Model file for the job. Use its own axes, mm. A direction names the side the tool comes from. Round coordinates to 2 decimals unless told otherwise and drop trailing zeros. Order: outer loops, then holes, each group sorted by start corner. A loop starts at its lowest first (then second) coordinate and runs counter-clockwise, first axis right, second up. Notation, with made-up numbers: (-28.75, 26.25) -> (-22.75, 26.25) arc R31 cw to (-22.75, 57.25) -> close; hole circle Ø10 at (-17, 9.25). An arc over 180 degrees is marked (long way). Answer as CSV lines item,"result".
```python
from build123d import *

# Parameters (mm, degrees)
SKETCH1_R             = 3
BOSS_EXTRUDE1_DEPTH   = 2
SKETCH2_R             = 3
BOSS_EXTRUDE2_DEPTH   = 2
SKETCH3_R             = 5
CUT_EXTRUDE1_DEPTH    = 38
BOSS_EXTRUDE3_DEPTH   = 35
CUT_EXTRUDE2_DEPTH    = 13
SKETCH6_R             = 3.5
CUT_EXTRUDE3_DEPTH    = 42
SKETCH7_W             = 6
SKETCH7_H             = 6
CUT_EXTRUDE4_DEPTH    = 5
BODY_MOVE_COPY1_ANGLE = 90
BODY_MOVE_COPY2_ANGLE = 45
BODY_MOVE_COPY3_ANGLE = 45
CUT_EXTRUDE5_DEPTH    = 10
BOSS_EXTRUDE4_START   = 1
BOSS_EXTRUDE4_DEPTH   = 1


with BuildPart() as part:
    # Sketch1 → Boss-Extrude1 (new body)
    with BuildSketch(Plane.XY):
        with BuildLine():
            Line((10, 0), (10, 25))
            Line((10, 25), (10, 25.027864045))
            ThreePointArc((10, 25.027864045), (10.597396767, 27.130788493), (12.211145618, 28.605572809))
            Line((12.211145618, 28.605572809), (15, 30))
            Line((15, 30), (15, 60))
            Line((15, 60), (-9.181612248, 3.962069729))
            ThreePointArc((-9.181612248, 3.962069729), (-2.022854113, -9.793266117), (10, 0))
        make_face()
        Circle(SKETCH1_R, mode=Mode.SUBTRACT)
    extrude(amount=BOSS_EXTRUDE1_DEPTH)


with BuildPart() as body_2:
    # Sketch2 → Boss-Extrude2 (new body)
    with BuildSketch(Plane.XY.offset(8)):
        with BuildLine():
            Line((10, 0), (10, 25.027864045))
            Line((10, 25.027864045), (10, 25.043361255))
            ThreePointArc((10, 25.043361255), (10.602103374, 27.153882167), (12.22714926, 28.629027198))
            Line((12.22714926, 28.629027198), (15, 30))
            Line((15, 30), (15, 60))
            Line((15, 60), (-9.181612248, 3.962069729))
            ThreePointArc((-9.181612248, 3.962069729), (-2.022854113, -9.793266117), (10, 0))
        make_face()
        Circle(SKETCH2_R, mode=Mode.SUBTRACT)
    extrude(amount=BOSS_EXTRUDE2_DEPTH)


with BuildPart() as cut_extrude1_tool:
    # Sketch3 → Cut-Extrude1 (new body)
    with BuildSketch(Plane(origin=(0, 60, 0), x_dir=(1, 0, 0), z_dir=(0, 1, 0))):
        with Locations((15, -5)):
            Circle(SKETCH3_R)
    extrude(amount=-CUT_EXTRUDE1_DEPTH)


with BuildPart() as part_1:
    add(part.part)

    # Cut-Extrude1: cut by cut_extrude1_tool
    add(cut_extrude1_tool.part, mode=Mode.SUBTRACT)



with BuildPart() as body_2_1:
    add(body_2.part)

    # Cut-Extrude1: cut by cut_extrude1_tool
    add(cut_extrude1_tool.part, mode=Mode.SUBTRACT)


with BuildPart() as part_2:
    add(part_1.part)

    add(body_2_1.part)  # Boss-Extrude3 merges body 2
    # Sketch4 → Boss-Extrude3 (add)
    with BuildSketch(Plane(origin=(0, 60, 0), x_dir=(1, 0, 0), z_dir=(0, 1, 0))):
        with BuildLine():
            ThreePointArc((15, 0), (10, -5), (15, -10))
            Line((15, -10), (15, 0))
        make_face()
        with BuildLine():
            Line((15, 0), (15, -10))
            ThreePointArc((15, -10), (18.535533906, -8.535533906), (20, -5))
            ThreePointArc((20, -5), (18.535533906, -1.464466094), (15, 0))
        make_face()
    extrude(amount=-BOSS_EXTRUDE3_DEPTH)

    # Sketch5 → Cut-Extrude2 (cut)
    with BuildSketch(Plane.XY):
        with BuildLine():
            Line((10, 25.027864045), (10, 25.043361255))
            ThreePointArc((10, 25.043361255), (10.602103374, 27.153882167), (12.22714926, 28.629027198))
            Line((12.22714926, 28.629027198), (15, 30))
            Line((15, 30), (20, 32.472135955))
            Line((20, 32.472135955), (20, 25))
            Line((20, 25), (20, 22.63115285))
            Line((20, 22.63115285), (10, 22.63115285))
            Line((10, 22.63115285), (10, 25.027864045))
        make_face()
    extrude(amount=CUT_EXTRUDE2_DEPTH, mode=Mode.SUBTRACT)

    # Sketch6 → Cut-Extrude3 (cut)
    with BuildSketch(Plane(origin=(0, 60, 0), x_dir=(1, 0, 0), z_dir=(0, 1, 0))):
        with Locations(Location((15, -5, 0), (0, 0, 270))):
            Circle(SKETCH6_R)
    extrude(amount=-CUT_EXTRUDE3_DEPTH, mode=Mode.SUBTRACT)

    # Sketch7 → Cut-Extrude4 (cut)
    with BuildSketch(Plane(origin=(0, 0, 0), x_dir=(-1, 0, 0), z_dir=(0, 0, -1))):
        Rectangle(SKETCH7_W, SKETCH7_H)
    extrude(amount=-CUT_EXTRUDE4_DEPTH, mode=Mode.SUBTRACT)


with BuildPart() as part_3:
    # Body-Move/Copy1: moved
    add(part_2.part.rotate(Axis((5, 0, 5), (0, 1, 0)), BODY_MOVE_COPY1_ANGLE))


with BuildPart() as part_4:
    # Body-Move/Copy2: moved
    add(part_3.part.rotate(Axis((5, 0, 5), (0, 1, 0)), BODY_MOVE_COPY2_ANGLE))


with BuildPart() as part_5:
    # Body-Move/Copy3: moved
    add(part_4.part.rotate(Axis((6.035533906, 0, 6.035533906), (0, 1, 0)), BODY_MOVE_COPY3_ANGLE))

    # Sketch8 → Cut-Extrude5 (cut)
    with BuildSketch(Plane(origin=(0, 0, 0), x_dir=(0, 0, -1), z_dir=(1, 0, 0))):
        Polygon((-3.035533906, 27.346279357), (-5.863961031, 30.174706482), (-9.035533906, 27.346279357), (-6.035533906, 25.043361255), align=None)
    extrude(amount=-CUT_EXTRUDE5_DEPTH, mode=Mode.SUBTRACT)

    # Sketch11 → Boss-Extrude4 (add)
    with BuildSketch(Plane(origin=(0, 60, 0), x_dir=(1, 0, 0), z_dir=(0, 1, 0)).offset(BOSS_EXTRUDE4_START)):
        with BuildLine():
            Line((-10.403869374, -5.535533906), (-10.403869374, -6.535533906))
            Line((-10.403869374, -6.535533906), (-8.893033803, -6.535533906))
            ThreePointArc((-8.893033803, -6.535533906), (-8.928932188, -6.035533906), (-8.893033803, -5.535533906))
            Line((-8.893033803, -5.535533906), (-10.403869374, -5.535533906))
        make_face()
    extrude(amount=-BOSS_EXTRUDE4_DEPTH)


solid = part_5.part
```
Q1. Saw through at C-C (y = -6). Write the cut outline in (x, z), plus the area to 3 significant figures.
Checks:
outline,"(1.57, 1.04) -> (17.57, 1.04) -> (17.57, 3.04) -> (1.57, 3.04) -> close; (1.57, 9.04) -> (17.57, 9.04) -> (17.57, 11.04) -> (1.57, 11.04) -> close"
area,"64.0 mm²"
Q2. Flat gauge pins, fed straight in: pin 1 (1.6 mm diameter, centred on y = 16, z = 2, fed in from -X); pin 2 (2 mm diameter, centred on x = 11, z = 10.5, fed in from +Y); pin 3 (1.6 mm diameter, centred on x = 8.5, z = 10, fed in from -Y). Where does each tip first touch, or does it go through?
Checks:
pin 1,"x = -0.43"
pin 2,"y = 24.25"
pin 3,"y = -10"
Q3. Saw through at B-B (y = 37.5). Write the cut outline in (x, z), plus the area to 3 significant figures.
Checks:
outline,"(-5.43, 1.04) -> (4.28, 1.04) -> (4.28, 3.04) -> (-1.43, 3.04) arc R5 ccw to (-1.43, 9.04) -> (4.28, 9.04) -> (4.28, 11.04) -> (-5.43, 11.04) arc R5 ccw to start; hole circle Ø7 at (-5.43, 6.04)"
area,"67.7 mm²"
Q4. Wall check: L1, parallel to Z at x = 5.5, y = 23.5; L2, parallel to Y at x = 9, z = 10; L3, parallel to X at y = 32.5, z = 7. Give the ranges that are in metal, low to high. Write a range as [from, to].
Checks:
L1,"[1.04, 3.04], [9.04, 11.04]"
L2,"[-9.98, -3], [3, 26.56]"
L3,"[-10.34, -8.79], [-2.06, -0.52]"
Q5. Tool access for faces 5 (the flat face through (6.493, 32.373, 10.05)), 6 (the flat face through (12.571, 0, 10)), 7 (the flat face through (6.493, 32.373, 2.05)), 8 (the flat face through (-1.39, 29.16, 7)), 9 (the flat face through (-0.429, 12, 2)): list every direction of +Z, -Z, +X, -X, +Y, -Y with a clear straight run to the whole face (end or side of a thin tool).
Checks:
face 5,"+Z, +X, +Y"
face 6,"+Z"
face 7,"-Z, +X, +Y"
face 8,"+X, -X, -Y"
face 9,"+Z, -Z, -X, -Y"
Q6. Saw through at A-A (x = 16.5). Write the cut outline in (y, z), plus the area to 3 significant figures.
Checks:
outline,"(-7.21, 1.04) -> (9.18, 1.04) -> (9.18, 3.04) -> (-7.21, 3.04) -> close; (-7.21, 9.04) -> (9.18, 9.04) -> (9.18, 11.04) -> (-7.21, 11.04) -> close"
area,"65.6 mm²"
Q7. Saw through at D-D (x = -4). Write the cut outline in (y, z), plus the area to 3 significant figures.
Checks:
outline,"(29.29, 1.04) -> (56.69, 1.04) -> (56.69, 1.24) -> (60, 1.24) -> (60, 2.84) -> (29.29, 2.84) -> close; (29.29, 9.23) -> (60, 9.23) -> (60, 10.83) -> (56.69, 10.83) -> (56.69, 11.04) -> (29.29, 11.04) -> close"
area,"109 mm²"
Q8. Mould opens along Z. For faces 1 (the flat face through (7, 18, 11.036)), 2 (the cylindrical face through (11.84, -9.74, 10.05)), 3 (the cylindrical face through (-0.43, 47.6, 6.15)), 4 (the flat face through (-1.42, 29.13, 4.82)) say: +Z half, -Z half, draft (parallel to the pull), parting line (faces both ways), or undercut.
Checks:
face 1,"+Z half"
face 2,"draft"
face 3,"undercut"
face 4,"undercut"
